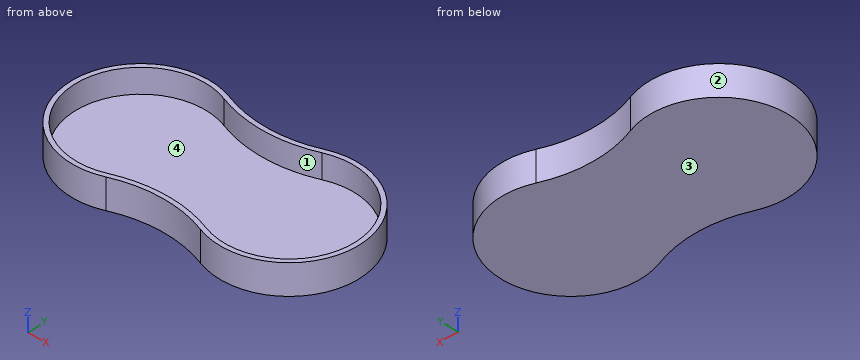
from build123d import *

# Parameters (mm, degrees)
BOSS_EXTRUDE1_DEPTH = 15
CUT_EXTRUDE2_DEPTH  = 12


with BuildPart() as part:
    # Sketch1 → Boss-Extrude1 (new body)
    with BuildSketch(Plane.XY):
        with BuildLine():
            ThreePointArc((-23.009618943, 32.5), (-71, 0), (-23.009618943, -32.5))
            ThreePointArc((-23.009618943, -32.5), (0, -28.07179677), (23.009618943, -32.5))
            ThreePointArc((23.009618943, -32.5), (71, 0), (23.009618943, 32.5))
            ThreePointArc((23.009618943, 32.5), (0, 28.07179677), (-23.009618943, 32.5))
        make_face()
    extrude(amount=BOSS_EXTRUDE1_DEPTH)

    # Sketch2 → Cut-Extrude2 (cut)
    with BuildSketch(Plane.XY.offset(15)):
        with BuildLine():
            ThreePointArc((-23.826157181, 30.457142857), (0, 25.87179677), (23.826157181, 30.457142857))
            ThreePointArc((23.826157181, 30.457142857), (68.8, 0), (23.826157181, -30.457142857))
            ThreePointArc((23.826157181, -30.457142857), (0, -25.87179677), (-23.826157181, -30.457142857))
            ThreePointArc((-23.826157181, -30.457142857), (-68.8, 0), (-23.826157181, 30.457142857))
        make_face()
    extrude(amount=-CUT_EXTRUDE2_DEPTH, mode=Mode.SUBTRACT)


solid = part.part
For this review, take the finished solid that the model builds, in its own axes (mm). Face numbers are marked on the shaded views. A direction names the side the tool comes from. Give positions to 0.01 mm unless a question says otherwise; leave off trailing zeros. Loops run counter-clockwise (first coordinate to the right, second up) from the corner with the lowest first, then second, coordinate; pieces in that order, holes last. Notation, with made-up numbers: M -14,16 L 18,16 A19 ccw 18,34 Z; hole C -20.5,69.25 d3. An arc over 180 degrees is marked long. Put each result on its own line as item: value. Start each with the question number.
(1) Add section B-B, the plane y = 0. Write out the cut boundary in (x, z), then the cut area to 3 significant figures.
(2) Add section C-C, the plane x = 36. Write out the cut boundary in (y, z), then the cut area to 3 significant figures.
(3) Wall thickness on L1, parallel to X at y = 0, z = 10.5; L2, parallel to Y at x = 36, z = 10.5; L3, parallel to X at y = 9.5, z = 4.5: over which ranges is each line inside the solid? List them lowest first.
(4) Machinability: for the marked faces 1 and 2, which of the approach directions +Z, -Z, +X, -X, +Y, -Y give a long, thin tool a straight path to every point of the face, cutting with its end or side? Answer none if there is none.
(5) The part is to be moulded in two halves that separate along X. For the marked faces 3 and 4, say which applies: +X half, -X half, draft (parallel to the pull), parting line (faces both ways), or undercut.
(6) Add section A-A, the plane z = 5.5. Write out the cut boundary in (x, y), then the cut area to 3 significant figures.
(7) For pin 1 (5 mm diameter, centred on x = -46.5, z = 4.5, fed in from -Y); pin 2 (2 mm diameter, centred on x = -54, y = -2.5, fed in from +Z); pin 3 (6 mm diameter, centred on x = 24.5, z = 6.5, fed in from +Y), all flat-tipped, find the tip position at first contact; note any pin that passes through.
Result:
1. outline: M -71,0 L 71,0 L 71,15 L 68.8,15 L 68.8,3 L -68.8,3 L -68.8,15 L -71,15 Z
1. area: 479 mm^2
2. outline: M -35,0 L 35,0 L 35,15 L 32.8,15 L 32.8,3 L -32.8,3 L -32.8,15 L -35,15 Z
2. area: 263 mm^2
3. L1: x = -71 to -68.8, 68.8 to 71
3. L2: y = -35 to -32.8, 32.8 to 35
3. L3: x = -69.69 to -67.39, 67.39 to 69.69
4. face 1: +Z
4. face 2: +Z, -Z
5. face 3: draft
5. face 4: undercut
6. outline: M -23.01,-32.5 A61.99 cw 23.01,-32.5 A35 ccw long 23.01,32.5 A61.99 cw -23.01,32.5 A35 ccw long Z; hole M -23.83,-30.46 A64.19 cw 23.83,-30.46 A32.8 ccw long 23.83,30.46 A64.19 cw -23.83,30.46 A32.8 ccw long Z
6. area: 793 mm^2
7. pin 1: stops at y = -34.07
7. pin 2: stops at z = 3
7. pin 3: stops at y = 33.95
